Input: part model. Units: mm. Frame: model coordinates. Give positions to 0.01 mm unless a question says otherwise; leave off trailing zeros. Order: outer loops, then holes, each group sorted by start corner. A loop starts at its lowest first (then second) coordinate and runs counter-clockwise, first axis right, second up.
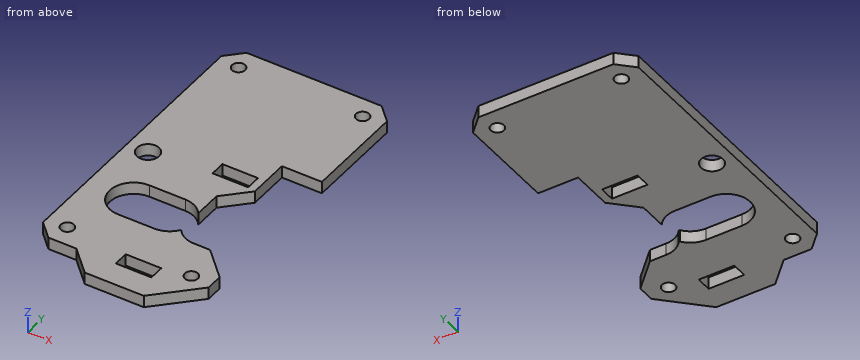
```python
from build123d import *

# Parameters (mm, degrees)
SKETCH1_R           = 1.65
SKETCH1_R_2         = 2.75
BOSS_EXTRUDE1_DEPTH = 3


with BuildPart() as part:
    # Sketch1 → Boss-Extrude1 (new body)
    with BuildSketch(Plane.XY):
        with BuildLine():
            Line((10.7, 26.7), (20.7, 26.7))
            Line((20.7, 26.7), (20.7, 51.73272542))
            Line((20.7, 51.73272542), (16.88272542, 55.55))
            Line((16.88272542, 55.55), (6.037050808, 55.55))
            Line((6.037050808, 55.55), (2.572949192, 55.55))
            Line((2.572949192, 55.55), (-16.88272542, 55.55))
            Line((-16.88272542, 55.55), (-20.7, 51.73272542))
            Line((-20.7, 51.73272542), (-20.7, 16.875735931))
            Line((-20.7, 16.875735931), (-20.7, -16.875735931))
            Line((-20.7, -16.875735931), (-16.875735931, -20.7))
            Line((-16.875735931, -20.7), (-9.875735931, -20.7))
            Line((-9.875735931, -20.7), (-3.875735931, -26.7))
            Line((-3.875735931, -26.7), (2.572949192, -26.7))
            Line((2.572949192, -26.7), (6.037050808, -26.7))
            Line((6.037050808, -26.7), (10.875735931, -26.7))
            Line((10.875735931, -26.7), (20.7, -16.875735931))
            Line((20.7, -16.875735931), (20.7, -12.624264069))
            Line((20.7, -12.624264069), (13.875735931, -5.8))
            Line((13.875735931, -5.8), (9.805, -5.8))
            ThreePointArc((9.805, -5.8), (7.212268524, -5.188231249), (5.166486047, -3.481980515))
            Line((5.166486047, -3.481980515), (4.88628813, -3.481980515))
            ThreePointArc((4.88628813, -3.481980515), (2.748464745, -5.333473685), (0, -6))
            Line((0, -6), (-9, -6))
            ThreePointArc((-9, -6), (-15, 0), (-9, 6))
            Line((-9, 6), (0, 6))
            ThreePointArc((0, 6), (2.748464745, 5.333473685), (4.88628813, 3.481980515))
            Line((4.88628813, 3.481980515), (4.88628813, 10.481980515))
            Line((4.88628813, 10.481980515), (10.7, 16.295692385))
            Line((10.7, 16.295692385), (10.7, 26.7))
        make_face()
        with Locations((-15.5, -15.5)):
            Circle(SKETCH1_R, mode=Mode.SUBTRACT)
        Polygon((6.037050808, -20.5), (2.572949192, -20.5), (-0.145, -20.5), (-0.145, -16.7), (8.755, -16.7), (8.755, -20.5), align=None, mode=Mode.SUBTRACT)
        with Locations((15.5, -15.5)):
            Circle(SKETCH1_R, mode=Mode.SUBTRACT)
        with Locations((-15.5, 15.5)):
            Circle(SKETCH1_R_2, mode=Mode.SUBTRACT)
        with Locations((-15.5, 50.35)):
            Circle(SKETCH1_R, mode=Mode.SUBTRACT)
        Polygon((-0.145, 20.5), (2.572949192, 20.5), (6.037050808, 20.5), (8.755, 20.5), (8.755, 16.7), (-0.145, 16.7), align=None, mode=Mode.SUBTRACT)
        with Locations((15.5, 50.35)):
            Circle(SKETCH1_R, mode=Mode.SUBTRACT)
    extrude(amount=BOSS_EXTRUDE1_DEPTH)


solid = part.part
```
1) Cut plane B-B (x = -5.5). Return the cut outline in (y, z), then the cut area to 3 significant figures.
2) Cut plane D-D (y = 15.5). Return the cut outline in (x, z), then the cut area to 3 significant figures.
3) Cut plane C-C (x = 15.5). Return the cut outline in (y, z).
4) Cut plane A-A (y = -15.5). Return the cut outline in (x, z), then the cut area to 3 significant figures.
5) First-contact query: P1, Ø0.9, axis at y = 19.5, z = 2, coming from the +X side. Flat tip, straight axial feed; report the tip coordinate or a pass-through.
6) Line query: probe 1 along Y at (x, z) = (-15.5, 0.95); probe 2 along X at (y, z) = (50.5, 2.2); probe 3 along Y at (x, z) = (15.5, 1.5). Output: solid intervals per line, ascending.
Geometry says:
1. outline: (-25.08, 0) - (-6, 0) - (-6, 3) - (-25.08, 3) - close; (6, 0) - (55.55, 0) - (55.55, 3) - (6, 3) - close
1. area: 206 mm2
2. outline: (-20.7, 0) - (-18.25, 0) - (-18.25, 3) - (-20.7, 3) - close; (-12.75, 0) - (9.9, 0) - (9.9, 3) - (-12.75, 3) - close
2. area: 75.3 mm2
3. outline: (-22.08, 0) - (-17.15, 0) - (-17.15, 3) - (-22.08, 3) - close; (-13.85, 0) - (-7.42, 0) - (-7.42, 3) - (-13.85, 3) - close; (26.7, 0) - (48.7, 0) - (48.7, 3) - (26.7, 3) - close; (52, 0) - (55.55, 0) - (55.55, 3) - (52, 3) - close
4. outline: (-20.7, 0) - (-17.15, 0) - (-17.15, 3) - (-20.7, 3) - close; (-13.85, 0) - (13.85, 0) - (13.85, 3) - (-13.85, 3) - close; (17.15, 0) - (20.7, 0) - (20.7, 3) - (17.15, 3) - close
4. area: 104 mm2
5. P1: stops at x = 10.7
6. probe 1: y = -20.7 to -17.15, -13.85 to 12.75, 18.25 to 48.7, 52 to 55.55
6. probe 2: x = -20.7 to -17.14, -13.86 to 13.86, 17.14 to 20.7
6. probe 3: y = -22.08 to -17.15, -13.85 to -7.42, 26.7 to 48.7, 52 to 55.55
